```python
from build123d import *

# Parameters (mm, degrees)
SKETCH1_W           = 80
SKETCH1_H           = 50
BOSS_EXTRUDE1_DEPTH = 5
SKETCH1_3_W         = 90
SKETCH1_3_H         = 4
BOSS_EXTRUDE2_DEPTH = 7.5
SKETCH1_4_R         = 5
CUT_EXTRUDE1_DEPTH  = 5


with BuildPart() as part:
    # Sketch1 → Boss-Extrude1 (new body)
    with BuildSketch(Plane(origin=(0, 0, 0), x_dir=(1, 0, 0), z_dir=(0, 1, 0))):
        Rectangle(SKETCH1_W, SKETCH1_H)
    extrude(amount=BOSS_EXTRUDE1_DEPTH)

    # Sketch1<3> → Boss-Extrude2 (add)
    with BuildSketch(Plane(origin=(0, 0, 0), x_dir=(1, 0, 0), z_dir=(0, 1, 0))):
        Rectangle(SKETCH1_3_W, SKETCH1_3_H)
        with Locations((0, -5)):
            Rectangle(SKETCH1_3_W, SKETCH1_3_H)
        with Locations((0, -10)):
            Rectangle(SKETCH1_3_W, SKETCH1_3_H)
    extrude(amount=BOSS_EXTRUDE2_DEPTH)

    # Sketch1<4> → Cut-Extrude1 (cut)
    with BuildSketch(Plane(origin=(0, 0, 0), x_dir=(1, 0, 0), z_dir=(0, 1, 0))):
        with Locations(Location((0, -17.5, 0), (0, 0, 90))):
            Circle(SKETCH1_4_R)
    extrude(amount=CUT_EXTRUDE1_DEPTH, mode=Mode.SUBTRACT)


solid = part.part
```
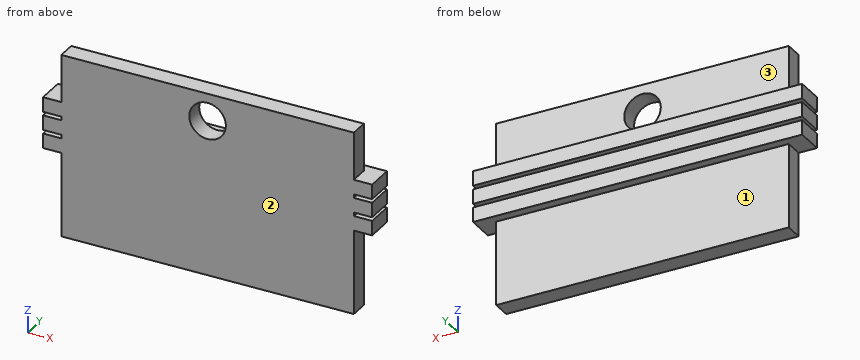
Input: part model. Units: mm. Frame: model coordinates. Face numbers are marked on the shaded views. A direction names the side the tool comes from. Coordinates: 2 decimals unless noted, no trailing zeros. Write each loop counter-clockwise with the first axis right and the second up, starting at its lowest first coordinate (ties: lowest second). Pieces come first, ordered by that corner, then holes.
1) Set-up query: the marked faces 1, 2 and 3. Return all of +Z, -Z, +X, -X, +Y, -Y with unobstructed straight access to the full face (end or side cutting, diameter ignored); none if empty.
2) Material intervals for line 1 along Z through (x, y) = (-38.5, 5.5); line 2 along X through (y, z) = (1.5, 17.5); line 3 along Y through (x, z) = (33, -11), sorted ascending.
3) Section B-B on x = 0. Output: boundary loops of the cut face in (y, z), and give its area (3 significant figures).
4) Section D-D on x = 39. Output: boundary loops of the cut face in (y, z), and give its area (3 significant figures).
5) Section A-A on y = 6. Output: boundary loops of the cut face in (x, z).
6) Section C-C on z = 17.5. Output: boundary loops of the cut face in (x, y), and give its area (3 significant figures).
7) Pin query (flat end, axial travel): pin 1 Ø0.5 at (x, z) = (4, 2.5) entering from +Y; pin 2 Ø1.5 at (y, z) = (3, -14.5) entering from +X; pin 3 Ø8 at (x, z) = (0, 17.5) entering from +Y. Return the tip coordinate at first contact, or that it passes through.
Check result:
1. face 1: -Z, +X, -X, +Y
1. face 2: +Z, -Z, +X, -X, -Y
1. face 3: +Z, +X, -X, +Y
2. line 1: z = -2 to 2, 3 to 7, 8 to 12
2. line 2: x = -40 to -5, 5 to 40
2. line 3: y = 0 to 5
3. outline: (0, -25) - (5, -25) - (5, -2) - (7.5, -2) - (7.5, 2) - (5, 2) - (5, 3) - (7.5, 3) - (7.5, 7) - (5, 7) - (5, 8) - (7.5, 8) - (7.5, 12) - (5, 12) - (5, 12.5) - (0, 12.5) - close; (0, 22.5) - (5, 22.5) - (5, 25) - (0, 25) - close
3. area: 230 mm2
4. outline: (0, -25) - (5, -25) - (5, -2) - (7.5, -2) - (7.5, 2) - (5, 2) - (5, 3) - (7.5, 3) - (7.5, 7) - (5, 7) - (5, 8) - (7.5, 8) - (7.5, 12) - (5, 12) - (5, 25) - (0, 25) - close
4. area: 280 mm2
5. outline: (-45, -2) - (45, -2) - (45, 2) - (-45, 2) - close; (-45, 3) - (45, 3) - (45, 7) - (-45, 7) - close; (-45, 8) - (45, 8) - (45, 12) - (-45, 12) - close
6. outline: (-40, 0) - (-5, 0) - (-5, 5) - (-40, 5) - close; (5, 0) - (40, 0) - (40, 5) - (5, 5) - close
6. area: 350 mm2
7. pin 1: stops at y = 5
7. pin 2: stops at x = 40
7. pin 3: passes through
